from build123d import *

# Parameters (mm, degrees)
SKETCH2_R           = 150
SKETCH2_R_2         = 5
BOSS_EXTRUDE1_DEPTH = 9
SKETCH3_R           = 150
BOSS_EXTRUDE2_DEPTH = 40
SKETCH9_R           = 144.906998713
CUT_EXTRUDE2_DEPTH  = 40
SKETCH11_W          = 33.774160464
SKETCH11_H          = 12.160705968
CUT_EXTRUDE9_DEPTH  = 40


with BuildPart() as part:
    # Sketch2 → Boss-Extrude1 (new body)
    with BuildSketch(Plane(origin=(0, 0, 0), x_dir=(1, 0, 0), z_dir=(0, 1, 0))):
        with Locations(Location((0, 0, 0), (0, 0, 270))):
            Circle(SKETCH2_R)
        with Locations(Location((0, 0, 0), (0, 0, 270))):
            Circle(SKETCH2_R_2, mode=Mode.SUBTRACT)
    extrude(amount=BOSS_EXTRUDE1_DEPTH)

    # Sketch3 → Boss-Extrude2 (add)
    with BuildSketch(Plane(origin=(0, 9, 0), x_dir=(1, 0, 0), z_dir=(0, 1, 0))):
        with Locations(Location((0, 0, 0), (0, 0, 270))):
            Circle(SKETCH3_R)
    extrude(amount=BOSS_EXTRUDE2_DEPTH)

    # Sketch9 → Cut-Extrude2 (cut)
    with BuildSketch(Plane(origin=(0, 49, 0), x_dir=(1, 0, 0), z_dir=(0, 1, 0))):
        with Locations(Location((0, 0, 0), (0, 0, 270))):
            Circle(SKETCH9_R)
    extrude(amount=-CUT_EXTRUDE2_DEPTH, mode=Mode.SUBTRACT)

    # Sketch11 → Cut-Extrude9 (cut)
    with BuildSketch(Plane(origin=(0, 49, 0), x_dir=(1, 0, 0), z_dir=(0, 1, 0))):
        with Locations((0, 150)):
            Rectangle(SKETCH11_W, SKETCH11_H)
    extrude(amount=-CUT_EXTRUDE9_DEPTH, mode=Mode.SUBTRACT)


solid = part.part
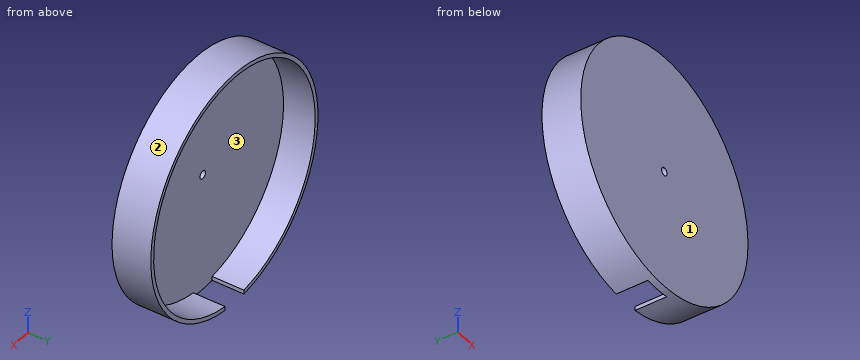
Part model, mm, in its own coordinate system. Face numbers are marked on the shaded views. Coordinates: 2 decimals unless noted, no trailing zeros. Order: outer loops, then holes, each group sorted by start corner. A loop starts at its lowest first (then second) coordinate and runs counter-clockwise, first axis right, second up. Notation, with made-up numbers: M 41.5,16.5 L 48.5,16.5 A8 ccw 48.5,30.5 Z; hole C 85,84.25 d4. An arc over 180 degrees is marked long. One line per question, with ' | ' between items.
Q1. Slice it at A-A (z = 0). Give the cut face in (x, y).
A:
outline: M -150,0 L -5,0 L -5,9 L -144.91,9 L -144.91,49 L -150,49 Z; M 5,0 L 150,0 L 150,49 L 144.91,49 L 144.91,9 L 5,9 Z
Q2. Slice it at D-D (y = 40). Give the cut face in (x, z), and give its area (3 significant figures).
A:
outline: M -16.89,-149.05 L -16.89,-143.92 A144.91 cw long 16.89,-143.92 L 16.89,-149.05 A150 ccw long Z | area: 4,550 mm^2
Q3. Two-plate mould, pull along Z, no slides. Class the marked faces 1, 2 and 3: +Z half, -Z half, draft (parallel to the pull), parting line (faces both ways), or undercut.
A:
face 1: draft | face 2: parting line | face 3: undercut
Q4. Slice it at C-C (z = -129). Give the cut face in (x, y), and give its area (3 significant figures).
A:
outline: M -76.54,0 L 76.54,0 L 76.54,49 L 66.01,49 L 66.01,9 L -66.01,9 L -66.01,49 L -76.54,49 Z | area: 2,220 mm^2
Q5. Drill centre lines: line 1 (X direction, y = 7, z = 0); line 2 (Y direction, x = 113.5, z = 61); line 3 (X direction, y = 41.5, z = -27.5). Where is each one in solid material? Low to high.
A:
line 1: x = -150 to -5, 5 to 150 | line 2: y = 0 to 9 | line 3: x = -147.46 to -142.27, 142.27 to 147.46
Q6. Slice it at B-B (x = 68). Give the cut face in (y, z), and give its area (3 significant figures).
A:
outline: M 0,-133.7 L 49,-133.7 L 49,-127.96 L 9,-127.96 L 9,127.96 L 49,127.96 L 49,133.7 L 0,133.7 Z | area: 2,870 mm^2
Q7. Pin check, flat tips, straight feed: P1, Ø4, axis at x = 22.5, y = 19.5, coming from the -Z side; P2, Ø1, axis at x = -27, z = 70, coming from the +Y side; P3, Ø6, axis at y = 21, z = 108.5, coming from the -X side; P4, Ø3, axis at x = 58, z = 22, coming from the -Y side. Stop position of each tip, or through.
A:
P1: stops at z = -148.59 | P2: stops at y = 9 | P3: stops at x = -106.63 | P4: stops at y = 0
